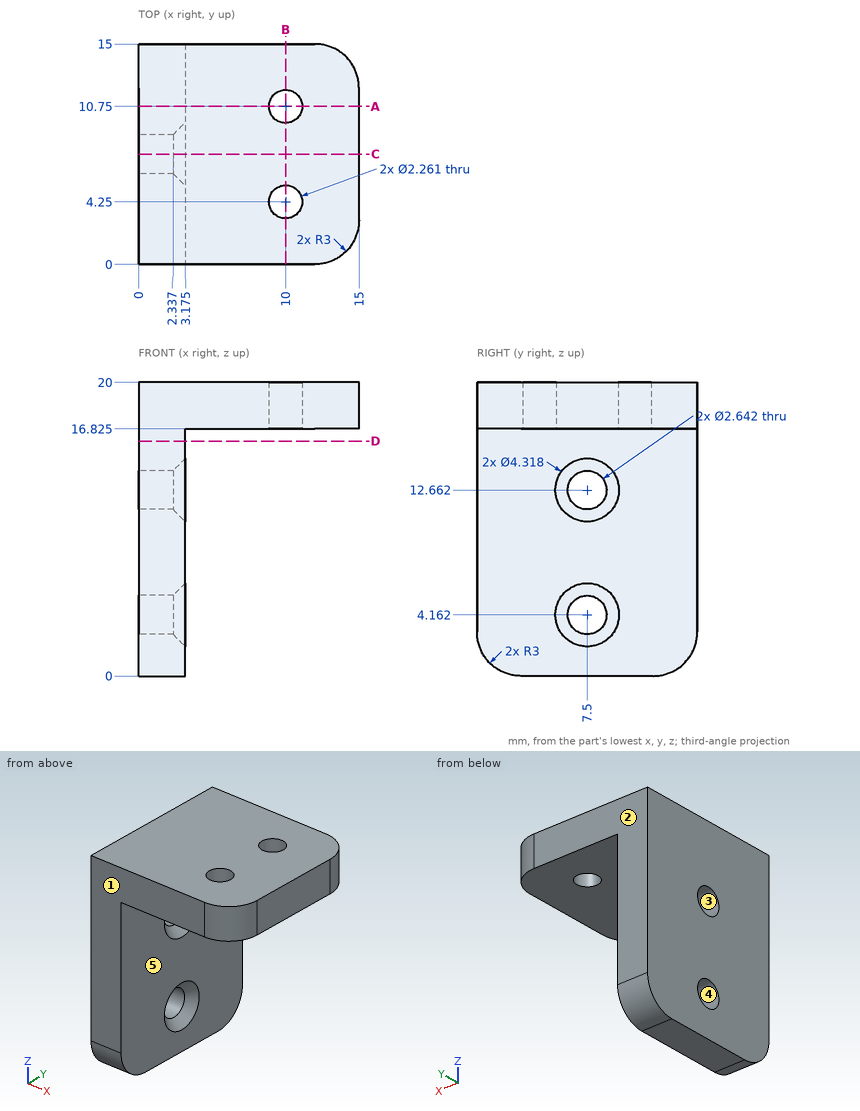
Check sheet for the drawn part. Datum: minimum x, y, z corner. Units: mm. A direction names the side the tool comes from. Coordinates: 2 decimals unless noted, no trailing zeros. Loops run counter-clockwise (first coordinate to the right, second up) from the corner with the lowest first, then second, coordinate; pieces in that order, holes last. Notation, with made-up numbers: (87.25, 46.5) -> (115.25, 46.5) arc R19 cw to (115.25, 51.5) -> close; hole circle Ø6 at (-14, 25). An arc over 180 degrees is marked (long way). Write each question's results on one line, items separated by ' | '.
Item 1: Section check A-A, the plane y = 10.75. Enter the section's corners in (x, z) (1 decimal).
Found:
outline: (0, 0) -> (3.2, 0) -> (3.2, 16.8) -> (8.9, 16.8) -> (8.9, 20) -> (0, 20) -> close; (11.1, 16.8) -> (15, 16.8) -> (15, 20) -> (11.1, 20) -> close
Item 2: Material ranges on L1, parallel to Z at x = 1.8, y = 7.5; L2, parallel to Y at x = 10, z = 18.6; L3, parallel to Y at x = 11, z = 19 (1 decimal), recorded low to high.
Found:
L1: z = 0 to 2.84, 5.48 to 11.34, 13.98 to 20 | L2: y = 0 to 3.12, 5.38 to 9.62, 11.88 to 15 | L3: y = 0 to 3.7, 4.8 to 10.2, 11.3 to 15
Item 3: Mould release check, pull along Y, two halves, no side actions. Record for the marked faces 1, 2 and 3: +Y half, -Y half, draft (parallel to the pull), parting line (faces both ways), or undercut.
Found:
face 1: -Y half | face 2: +Y half | face 3: undercut
Item 4: Section check C-C, the plane y = 7.5. Enter the section's corners in (x, z) (1 decimal).
Found:
outline: (0, 0) -> (3.2, 0) -> (3.2, 2) -> (2.3, 2.8) -> (0, 2.8) -> close; (0, 5.5) -> (2.3, 5.5) -> (3.2, 6.3) -> (3.2, 10.5) -> (2.3, 11.3) -> (0, 11.3) -> close; (0, 14) -> (2.3, 14) -> (3.2, 14.8) -> (3.2, 16.8) -> (15, 16.8) -> (15, 20) -> (0, 20) -> close
Item 5: Section check D-D, the plane z = 16. Enter the section's corners in (x, y) (1 decimal).
Found:
outline: (0, 0) -> (3.2, 0) -> (3.2, 15) -> (0, 15) -> close
Item 6: Tool access check on the marked faces 4 and 5. Record the directions out of +Z, -Z, +X, -X, +Y, -Y that give a thin tool (end or side, any length) a straight path to the whole face; none if there is none.
Found:
face 4: +X, -X | face 5: -Z, +X, +Y, -Y
Item 7: Section check B-B, the plane x = 10. Enter the section's corners in (y, z) (1 decimal).
Found:
outline: (0, 16.8) -> (3.1, 16.8) -> (3.1, 20) -> (0, 20) -> close; (5.4, 16.8) -> (9.6, 16.8) -> (9.6, 20) -> (5.4, 20) -> close; (11.9, 16.8) -> (15, 16.8) -> (15, 20) -> (11.9, 20) -> close
Item 8: Gauge pin test, flat ends, axial feed: pin 1 (3.5 mm diameter, centred on x = 11, y = 9, fed in from -Z) (1 decimal); pin 2 (1.5 mm diameter, centred on x = 10, z = 16, fed in from +Y); pin 3 (4 mm diameter, centred on y = 7.5, z = 4.16, fed in from +X); pin 4 (5 mm diameter, centred on y = 10, z = 17, fed in from -X). Record the tip position at first contact, or that the pin passes through.
Found:
pin 1: stops at z = 16.8 | pin 2: passes through | pin 3: stops at x = 3.02 | pin 4: stops at x = 0
